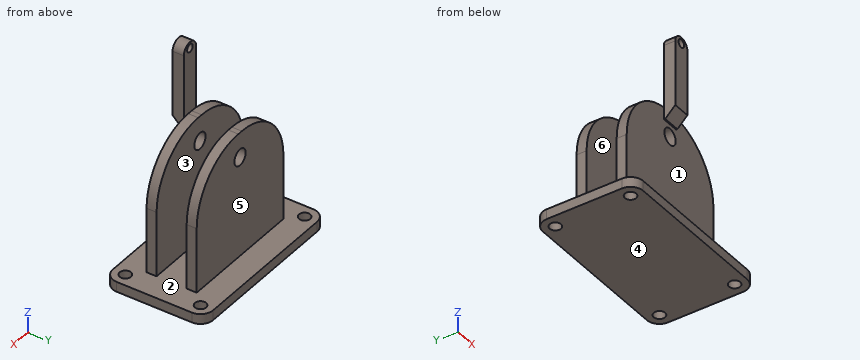
```python
from build123d import *

# Parameters (mm, degrees)
SKETCH_W        = 70
SKETCH_H        = 40
PAD_DEPTH       = 4
FILLET_R        = 5
SKETCH001_R     = 2.25
POCKET_DEPTH    = 5
SKETCH002_W     = 50
SKETCH002_H     = 4
PAD001_DEPTH    = 50
SKETCH003_R     = 3.25
POCKET001_DEPTH = 30.001
FILLET001_R     = 24
PAD004_DEPTH    = 4.5
CHAMFER_SIZE    = 4
SKETCH007_R     = 1.6
POCKET002_DEPTH = 4.5


with BuildPart() as part:
    # Sketch → Pad (new body)
    with BuildSketch(Plane.XY):
        Rectangle(SKETCH_W, SKETCH_H)
    extrude(amount=PAD_DEPTH)

    # Fillet
    fillet_edges = [part.edges().sort_by_distance(p)[0] for p in [
        (35, -20, 2),
        (35, 20, 2),
        (-35, -20, 2),
        (-35, 20, 2),
    ]]
    fillet(fillet_edges, radius=FILLET_R)

    # Sketch001 (on Face5 of Fillet) → Pocket (cut)
    with BuildSketch(Plane.XY.offset(4)):
        with Locations((-30, 15)):
            Circle(SKETCH001_R)
        with Locations((30, 15)):
            Circle(SKETCH001_R)
        with Locations((30, -15)):
            Circle(SKETCH001_R)
        with Locations((-30, -15)):
            Circle(SKETCH001_R)
    extrude(amount=-POCKET_DEPTH, mode=Mode.SUBTRACT)

    # Sketch002 (on Face5 of Pocket) → Pad001 (join)
    with BuildSketch(Plane.XY.offset(4)):
        with Locations((0, 8)):
            Rectangle(SKETCH002_W, SKETCH002_H)
        with Locations((0, -8)):
            Rectangle(SKETCH002_W, SKETCH002_H)
    extrude(amount=PAD001_DEPTH)

    # Sketch003 (on Face21 of Pad001) → Pocket001 (cut, through all)
    with BuildSketch(Plane.XZ.offset(10)):
        with Locations((0, 44)):
            Circle(SKETCH003_R)
    extrude(amount=-POCKET001_DEPTH, mode=Mode.SUBTRACT)

    # Fillet001
    fillet001_edges = [part.edges().sort_by_distance(p)[0] for p in [
        (-25, 8, 54),
        (-25, -8, 54),
        (25, 8, 54),
        (25, -8, 54),
    ]]
    fillet(fillet001_edges, radius=FILLET001_R)

    # Sketch006 (on Face21 of Fillet001) → Pad004 (join)
    with BuildSketch(Plane.XZ.offset(10)):
        with BuildLine():
            Line((3.5, 49), (-3.5, 49))
            Line((-3.5, 79), (-3.5, 49))
            ThreePointArc((3.5, 79), (0, 82.5), (-3.5, 79))
            Line((3.5, 49), (3.5, 79))
        make_face()
    extrude(amount=PAD004_DEPTH)

    # Chamfer
    chamfer_edges = [part.edges().sort_by_distance(p)[0] for p in [
        (0, -14.5, 49),
    ]]
    chamfer(chamfer_edges, length=CHAMFER_SIZE)

    # Sketch007 (on Face5 of Chamfer) → Pocket002 (cut)
    with BuildSketch(Plane.XZ.offset(14.5)):
        with Locations((0, 80)):
            Circle(SKETCH007_R)
    extrude(amount=-POCKET002_DEPTH, mode=Mode.SUBTRACT)


solid = part.part
```
Verification items for the finished model (mm, model axes). Face numbers are marked on the shaded views. A direction names the side the tool comes from. Coordinates: 2 decimals unless noted, no trailing zeros. Loops run counter-clockwise (first coordinate to the right, second up) from the corner with the lowest first, then second, coordinate; pieces in that order, holes last. Notation, with made-up numbers: (71, 22) -> (91, 22) arc R21 ccw to (91, 59) -> close; hole circle Ø10 at (67, 46.25). An arc over 180 degrees is marked (long way). Put each result on its own line as item: value.
1. Section check B-B, the plane z = 80. Record the boundary of the cut face in (x, y), then the cut area to 3 significant figures.
Result set:
outline: (-3.35, -14.5) -> (-1.6, -14.5) -> (-1.6, -10) -> (-3.35, -10) -> close; (1.6, -14.5) -> (3.35, -14.5) -> (3.35, -10) -> (1.6, -10) -> close
area: 15.8 mm^2
2. Tool access check on the marked faces 5 and 6. Record the directions out of +Z, -Z, +X, -X, +Y, -Y that give a thin tool (end or side, any length) a straight path to the whole face; none if there is none.
Result set:
face 5: +Z, +X, -X, +Y
face 6: +Z, +X, -X
3. Section check A-A, the plane y = -9. Record the boundary of the cut face in (x, z), then the cut area to 3 significant figures.
Result set:
outline: (-35, 0) -> (35, 0) -> (35, 4) -> (25, 4) -> (25, 30) arc R24 ccw to (1, 54) -> (-1, 54) arc R24 ccw to (-25, 30) -> (-25, 4) -> (-35, 4) -> close; hole circle Ø6.5 at (0, 44)
area: 2,500 mm^2
4. Thickness scan on line 1 (Y direction, x = -30, z = 2); line 2 (Y direction, x = 20.5, z = 29); line 3 (Z direction, x = 0, y = -11.5). Record the ranges inside material, lowest first.
Result set:
line 1: y = -20 to -17.25, -12.75 to 12.75, 17.25 to 20
line 2: y = -10 to -6, 6 to 10
line 3: z = 0 to 4, 50 to 78.4, 81.6 to 82.5
5. Section check C-C, the plane x = -12.5. Record the boundary of the cut face in (y, z).
Result set:
outline: (-20, 0) -> (20, 0) -> (20, 4) -> (10, 4) -> (10, 51.07) -> (6, 51.07) -> (6, 4) -> (-6, 4) -> (-6, 51.07) -> (-10, 51.07) -> (-10, 4) -> (-20, 4) -> close
6. Mould release check, pull along Y, two halves, no side actions. Record for the marked faces 1, 2, 3 and 4: pulls with the +Y half, pulls with the -Y half, needs draft (parallel to the pull), parting line crosses it, or undercut.
Result set:
face 1: pulls with the -Y half
face 2: undercut
face 3: undercut
face 4: needs draft
7. Section check D-D, the plane z = 68.5. Record the boundary of the cut face in (x, y), then the cut area to 3 significant figures.
Result set:
outline: (-3.5, -14.5) -> (3.5, -14.5) -> (3.5, -10) -> (-3.5, -10) -> close
area: 31.5 mm^2
8. Gauge pin test, flat ends, axial feed: P1, Ø1, axis at y = -13.5, z = 61, coming from the -X side; P2, Ø5, axis at x = 7, z = 43.5, coming from the -Y side; P3, Ø3.5, axis at x = -30, y = -15, coming from the -Z side; P4, Ø0.6, axis at x = 0.5, y = 7.5, coming from the +Z side. Record the tip position at first contact, or that the pin passes through.
Result set:
P1: stops at x = -3.5
P2: stops at y = -10
P3: passes through
P4: stops at z = 54
